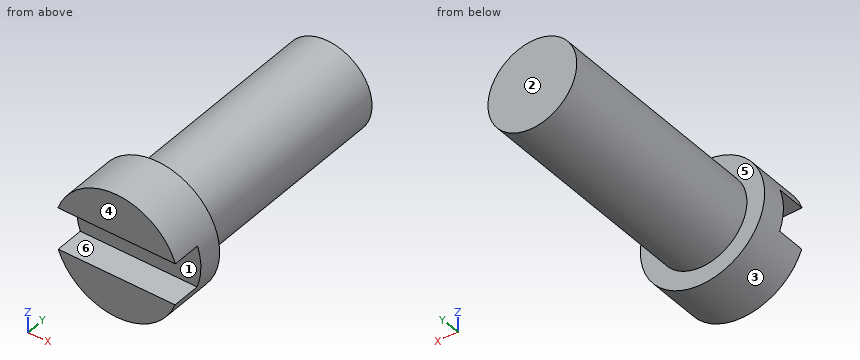
Autodesk Inventor part; units mm, degrees
ref_plane "YZ Plane" through (0, 0, 0) normal (1, 0, 0) x (0, 1, 0)
ref_plane "XZ Plane" through (0, 0, 0) normal (0, 1, 0) x (-1, 0, 0)
ref_plane "XY Plane" through (0, 0, 0) normal (0, 0, 1) x (1, 0, 0)
sketch "Esboço1" plane through (0, 0, 0) normal (0, 1, 0) x (-1, 0, 0)
  circle A0 centre (0, 0) radius 2.8
  dimension "d0" = 5.6
extrude "Extrusão1" add sketch "Esboço1" along normal blind 2.4
sketch "Esboço2" plane through (0, 0, 0) normal (1, 0, 0) x (0, 1, 0)
  line L0 (0, 0.9185) -> (1.2961, 0.9185)
  line L1 (1.2961, 0.9185) -> (1.2961, -0.9611)
  line L2 (1.2961, -0.9611) -> (0, -0.9611)
  line L3 (0, -0.9611) -> (0, 0.9185)
  point P0 (0, 0)
extrude "Extrusão2" cut sketch "Esboço2" along normal through all both and the other way through all
sketch "Esboço3" plane through (0, 2.4, 0) normal (0, 1, 0) x (1, 0, 0)
  circle A0 centre (0, 0) radius 2.8
  circle A1 centre (0, 0) radius 2
  dimension "d5" = 4
extrude "Extrusão3" add sketch "Esboço3" along normal blind 10 contours A1
thread "Rosca1"
properties part number "Parafuso-M4-10"
The listing builds one solid part. Answer for the finished solid, in the listing's coordinates (mm). Face numbers are marked on the shaded views. A direction names the side the tool comes from. Coordinates: 2 decimals unless noted, no trailing zeros. Loops run counter-clockwise (first coordinate to the right, second up) from the corner with the lowest first, then second, coordinate; pieces in that order, holes last. Notation, with made-up numbers: (0.5, 28.5) - (28.5, 28.5) arc R27 ccw to (28.5, 65.5) - close; hole circle Ø5 at (81.25, -13). An arc over 180 degrees is marked (long way). Use a Markdown table: item, result. Add a question column.
1) Given pin 1 (3 mm diameter, centred on y = 5.5, z = -0.5, fed in from -X); pin 2 (1 mm diameter, centred on x = -1, y = 1, fed in from -Z) (3 decimals); pin 3 (0.9 mm diameter, centred on x = -0.5, z = 0, fed in from -Y), each flat-ended and moving along its own axis, determine where each tip first touches the part or whether it passes through.
2) The part is cut by section B-B, the plane x = 0. Give the vertices of the cut face in (y, z).
3) The part is cut by section C-C, the plane y = 9.5. Give the vertices of the cut face in (x, z), and give its area (3 significant figures).
4) The mould has two halves that part along Z. Classify the marked faces 1, 2 and 3: released by +Z, released by -Z, zero draft, split by the parting line, or undercut.
5) The part is cut by section D-D, the plane x = 1.1. Give the vertices of the cut face in (y, z).
6) Find the intervals of material crossed by line 1 (Y direction, x = -0.8, z = 0.35); line 2 (Z direction, x = 0.1, y = 5.25); line 3 (Y direction, x = -1.5, z = -1.85), in increasing order.
7) For the marked faces 4, 5 and 6, determine the directions among +Z, -Z, +X, -X, +Y, -Y from which every point of the face is accessible in a straight line to the end or side of a thin tool.
8) The part is cut by section A-A, the plane z = 0. Give the vertices of the cut face in (x, y).
Here are the results:
| question | item | result |
|---|---|---|
| 1 | pin 1 | stops at x = -2 |
| 1 | pin 2 | stops at z = -2.755 |
| 1 | pin 3 | stops at y = 1.3 |
| 2 | outline | (0, -2.8) - (2.4, -2.8) - (2.4, -2) - (12.4, -2) - (12.4, 2) - (2.4, 2) - (2.4, 2.8) - (0, 2.8) - (0, 0.92) - (1.3, 0.92) - (1.3, -0.96) - (0, -0.96) - close |
| 3 | outline | circle Ø4 at (0, 0) |
| 3 | area | 12.6 mm^2 |
| 4 | face 1 | undercut |
| 4 | face 2 | zero draft |
| 4 | face 3 | split by the parting line |
| 5 | outline | (0, -2.57) - (2.4, -2.57) - (2.4, -1.67) - (12.4, -1.67) - (12.4, 1.67) - (2.4, 1.67) - (2.4, 2.57) - (0, 2.57) - (0, 0.92) - (1.3, 0.92) - (1.3, -0.96) - (0, -0.96) - close |
| 6 | line 1 | y = 1.3 to 12.4 |
| 6 | line 2 | z = -2 to 2 |
| 6 | line 3 | y = 0 to 2.4 |
| 7 | face 4 | +Z, -Z, +X, -X, -Y |
| 7 | face 5 | +Y |
| 7 | face 6 | +X, -X, -Y |
| 8 | outline | (-2.8, 1.3) - (2.8, 1.3) - (2.8, 2.4) - (2, 2.4) - (2, 12.4) - (-2, 12.4) - (-2, 2.4) - (-2.8, 2.4) - close |
